Work out the finished part from the listing and answer in its coordinate system (mm). Face numbers are marked on the shaded views. Give positions to 0.01 mm unless a question says otherwise; leave off trailing zeros. Loops run counter-clockwise (first coordinate to the right, second up) from the corner with the lowest first, then second, coordinate; pieces in that order, holes last. Notation, with made-up numbers: (76, 21.5) - (110, 21.5) arc R12 ccw to (110, 27.5) - close; hole circle Ø4 at (41.25, 81). An arc over 180 degrees is marked (long way). One line per item, written item: value.
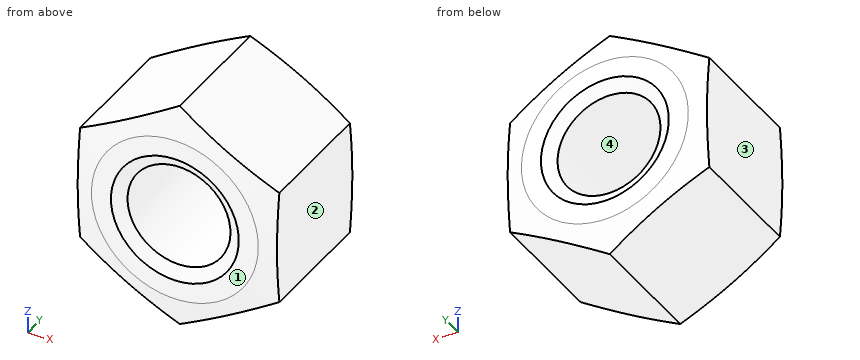
Solid Edge part; units mm, degrees
sketch "Sketch1" plane through (0, 0, 0) normal (0, -1, 0) x (1, 0, 0)
  line L0 (4, 2.3094) -> (0, 4.6188)
  line L1 (0, 4.6188) -> (-4, 2.3094)
  line L2 (-4, 2.3094) -> (-4, -2.3094)
  line L3 (-4, -2.3094) -> (0, -4.6188)
  line L4 (0, -4.6188) -> (4, -2.3094)
  line L5 (4, -2.3094) -> (4, 2.3094)
extrude "Protrusion1" add sketch "Sketch1" along normal mid plane 5.6
sketch "Sketch2" plane through (0, 0, 0) normal (1, 0, 0) x (0, 1, 0)
  line L0 (-2.8, 3.35) -> (-2.46, 4.6188)
revolve "RevolvedCutout1" cut sketch "Sketch2" angle 360 about axis through (0, 0, 0) along (0, -1, 0) material side at (0, -2.6783, 3.9973)
mirror "Mirror1" about plane through (0, 0, 0) normal (0, -1, 0) of "RevolvedCutout1"
hole "孔_7" at (0, -2.8, 0) direction (0, 1, 0) diameter 4.134 end up to next start chamfer 0.5 start chamfer angle 60 end chamfer 0.5 end chamfer angle 60
properties part number "N2611-1312" material "钢"
1. Section A-A (z = 0) is taken. Write down the section's boundary in (x, y).
Output:
outline: (-4, -2.63) - (-3.35, -2.8) - (-2.57, -2.8) - (-2.07, -2.51) - (-2.07, 2.51) - (-2.57, 2.8) - (-3.35, 2.8) - (-4, 2.63) - close; (2.07, -2.51) - (2.57, -2.8) - (3.35, -2.8) - (4, -2.63) - (4, 2.63) - (3.35, 2.8) - (2.57, 2.8) - (2.07, 2.51) - close
2. The mould has two halves that part along X. Classify the marked faces 1, 2, 3 and 4: released by +X, released by -X, zero draft, split by the parting line, or undercut.
Output:
face 1: zero draft
face 2: released by +X
face 3: released by -X
face 4: undercut
3. Section B-B (y = -1.1) is taken. Write down the section's boundary in (x, z).
Output:
outline: (-4, -2.31) - (0, -4.62) - (4, -2.31) - (4, 2.31) - (0, 4.62) - (-4, 2.31) - close; hole circle Ø4.13 at (0, 0)
4. Find the intervals of material crossed by line 1 along X through (y, z) = (0.1, 0); line 2 along Z through (x, y) = (-0.25, -0.55); line 3 along Z through (x, y) = (-1.75, 1.25), in increasing order.
Output:
line 1: x = -4 to -2.07, 2.07 to 4
line 2: z = -4.47 to -2.05, 2.05 to 4.47
line 3: z = -3.61 to -1.1, 1.1 to 3.61
